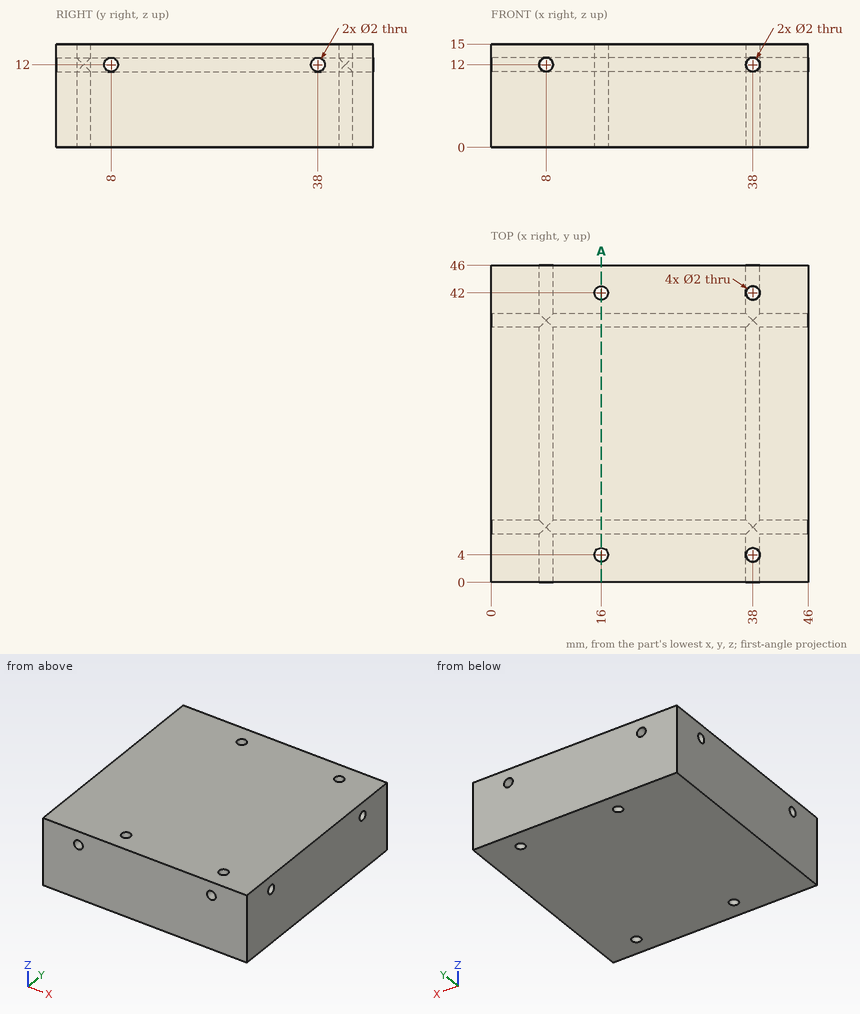
Can you work these out from the drawing? Everything is in mm from the part's minimum corner. Round coordinates to 2 decimals unless told otherwise and drop trailing zeros. Loops run counter-clockwise (first coordinate to the right, second up) from the corner with the lowest first, then second, coordinate; pieces in that order, holes last. Notation, with made-up numbers: (44, 5.25) - (101, 5.25) arc R27 ccw to (101, 33.25) - close; hole circle Ø5 at (-27, -16). An arc over 180 degrees is marked (long way). Answer in a Markdown table with one row per item. Add a question column.
(1) If we section it at A-A (x = 16): Please give me the cut outline in (y, z), plus the area to 3 significant figures.
(2) I'm going to push a flat-ended pin straight in: pin 1 (1.8 mm diameter, centred on y = 38, z = 12, fed in from -X). Where does the tip first touch, or does it pass through?
(3) I need wall thicknesses on line 1 along Y through (x, z) = (38, 5); line 2 along X through (y, z) = (4, 5.75); line 3 along X through (y, z) = (29, 12). Which ranges of each line are inside material? Lowest first, please.
Model answer:
| question | item | result |
|---|---|---|
| 1 | outline | (0, 0) - (3, 0) - (3, 15) - (0, 15) - close; (5, 0) - (41, 0) - (41, 15) - (5, 15) - close; (43, 0) - (46, 0) - (46, 15) - (43, 15) - close; hole circle Ø2 at (8, 12); hole circle Ø2 at (38, 12) |
| 1 | area | 624 mm² |
| 2 | pin 1 | passes through |
| 3 | line 1 | y = 0 to 3, 5 to 41, 43 to 46 |
| 3 | line 2 | x = 0 to 15, 17 to 37, 39 to 46 |
| 3 | line 3 | x = 0 to 7, 9 to 37, 39 to 46 |
